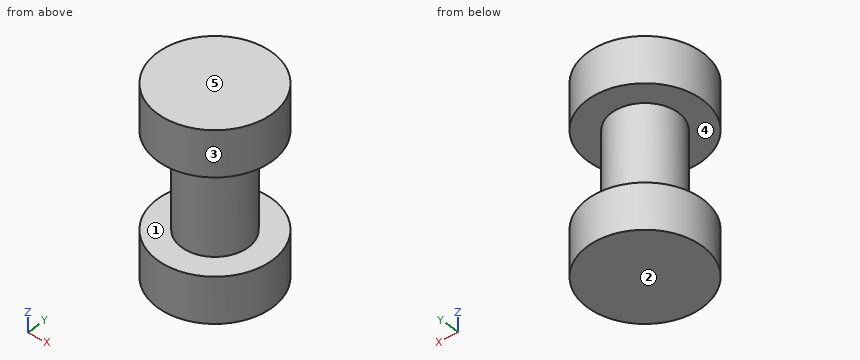
```python
from build123d import *

# Parameters (mm, degrees)
SKETCH1_R           = 12.5
BOSS_EXTRUDE1_DEPTH = 10
SKETCH3_R           = 7.25
BOSS_EXTRUDE2_DEPTH = 21
SKETCH4_R           = 12.5
BOSS_EXTRUDE3_DEPTH = 10


with BuildPart() as part:
    # Sketch1 → Boss-Extrude1 (new body)
    with BuildSketch(Plane.XY):
        Circle(SKETCH1_R)
    extrude(amount=BOSS_EXTRUDE1_DEPTH)

    # Sketch3 → Boss-Extrude2 (add)
    with BuildSketch(Plane.XY.offset(10)):
        with Locations(Location((0, 0, 0), (0, 0, 180))):
            Circle(SKETCH3_R)
    extrude(amount=BOSS_EXTRUDE2_DEPTH)

    # Sketch4 → Boss-Extrude3 (add)
    with BuildSketch(Plane.XY.offset(31)):
        Circle(SKETCH4_R)
    extrude(amount=BOSS_EXTRUDE3_DEPTH)


solid = part.part
```
Geometry check sheet. Reference: the model listing, model coordinates, mm. Face numbers are marked on the shaded views. A direction names the side the tool comes from. Round coordinates to 2 decimals unless told otherwise and drop trailing zeros. Order: outer loops, then holes, each group sorted by start corner. A loop starts at its lowest first (then second) coordinate and runs counter-clockwise, first axis right, second up. Notation, with made-up numbers: M 23.5,77 L 48.5,77 A24 cw 48.5,110 Z; hole C 71.5,-8.75 d8. An arc over 180 degrees is marked long. Answer as CSV lines item,"result".
1) Sectioned sample at B-B on x = 5.75. Record the cut outline in (y, z).
Entries:
outline,"M -11.1,0 L 11.1,0 L 11.1,10 L 4.42,10 L 4.42,31 L 11.1,31 L 11.1,41 L -11.1,41 L -11.1,31 L -4.42,31 L -4.42,10 L -11.1,10 Z"
2) Gauge pin test, flat ends, axial feed: pin 1 Ø1.5 at (y, z) = (7, 6) entering from +X; pin 2 Ø6 at (y, z) = (5.5, 33.5) entering from +X; pin 3 Ø8 at (x, y) = (-1.5, -8.5) entering from -Z; pin 4 Ø4 at (x, z) = (3.5, 19.5) entering from -Y. Record the tip position at first contact, or that the pin passes through.
Entries:
pin 1,"x = 10.83"
pin 2,"x = 12.25"
pin 3,"z = 0"
pin 4,"y = -7.09"
3) Sectioned sample at D-D on z = 9.5. Record the cut outline in (x, y), and give its area (3 significant figures).
Entries:
outline,"C 0,0 d25"
area,"491 mm2"
4) Mould release check, pull along Z, two halves, no side actions. Record for the marked faces 1, 2 and 3: +Z half, -Z half, draft (parallel to the pull), parting line (faces both ways), or undercut.
Entries:
face 1,"undercut"
face 2,"-Z half"
face 3,"draft"
5) Thickness scan on probe 1 along Z at (x, y) = (-7, -2.5); probe 2 along Y at (x, z) = (0.5, 3); probe 3 along Y at (x, z) = (-5.75, 34.5). Record the ranges inside material, lowest first. Write a range as [from, to].
Entries:
probe 1,"[0, 10], [31, 41]"
probe 2,"[-12.49, 12.49]"
probe 3,"[-11.1, 11.1]"
6) Sectioned sample at C-C on y = 0. Record the cut outline in (x, z), and give its area (4 significant figures).
Entries:
outline,"M -12.5,0 L 12.5,0 L 12.5,10 L 7.25,10 L 7.25,31 L 12.5,31 L 12.5,41 L -12.5,41 L -12.5,31 L -7.25,31 L -7.25,10 L -12.5,10 Z"
area,"804.5 mm2"
7) Sectioned sample at A-A on y = -8.25. Record the cut outline in (x, z), and give its area (3 significant figures).
Entries:
outline,"M -9.39,0 L 9.39,0 L 9.39,10 L -9.39,10 Z; M -9.39,31 L 9.39,31 L 9.39,41 L -9.39,41 Z"
area,"376 mm2"
8) Tool access check on the marked faces 4 and 5. Record the directions out of +Z, -Z, +X, -X, +Y, -Y that give a thin tool (end or side, any length) a straight path to the whole face; none if there is none.
Entries:
face 4,"none"
face 5,"+Z, +X, -X, +Y, -Y"
